```python
from build123d import *

# Parameters (mm, degrees)
SKETCH1_R           = 17.5
BOSS_EXTRUDE1_DEPTH = 3.5
CHAMFER1_SIZE       = 0.5
CUT_EXTRUDE1_DEPTH  = 1
SKETCH4_R           = 15.75
CUT_EXTRUDE2_DEPTH  = 1.5
FILLET1_R           = 1
THREAD1_PITCH       = 0.56


with BuildPart() as part:
    # Sketch1 → Boss-Extrude1 (new body)
    with BuildSketch(Plane(origin=(0, 0, 0), x_dir=(1, 0, 0), z_dir=(0, 1, 0))):
        with Locations(Location((0, 0, 0), (0, 0, 270))):
            Circle(SKETCH1_R)
    extrude(amount=BOSS_EXTRUDE1_DEPTH)

    # Chamfer1
    chamfer1_edges = [part.edges().sort_by_distance(p)[0] for p in [
        (0, 3.5, -17.5),
    ]]
    chamfer(chamfer1_edges, length=CHAMFER1_SIZE)

    # Sketch3 → Cut-Extrude1 (cut)
    with BuildSketch(Plane(origin=(0, 3.5, 0), x_dir=(1, 0, 0), z_dir=(0, 1, 0))):
        with BuildLine():
            Line((14.163644775, 9.216614608), (14.700580525, 9.526614608))
            ThreePointArc((14.700580525, 9.526614608), (15.170616014, 8.75875924), (15.600580525, 7.967768881))
            Line((15.600580525, 7.967768881), (15.063644775, 7.657768881))
            ThreePointArc((15.063644775, 7.657768881), (14.98776287, 7.647778839), (14.927042235, 7.694371422))
            Line((14.927042235, 7.694371422), (14.127042235, 9.080012068))
            ThreePointArc((14.127042235, 9.080012068), (14.117052192, 9.155893972), (14.163644775, 9.216614608))
        make_face()
        with BuildLine():
            Line((-0.8, 16.774383489), (0.8, 16.774383489))
            ThreePointArc((0.8, 16.774383489), (0.870710678, 16.803672811), (0.9, 16.874383489))
            Line((0.9, 16.874383489), (0.9, 17.494383489))
            ThreePointArc((0.9, 17.494383489), (0, 17.517518479), (-0.9, 17.494383489))
            Line((-0.9, 17.494383489), (-0.9, 16.874383489))
            ThreePointArc((-0.9, 16.874383489), (-0.870710678, 16.803672811), (-0.8, 16.774383489))
        make_face()
        with BuildLine():
            Line((15.063644775, -7.657768881), (15.600580525, -7.967768881))
            ThreePointArc((15.600580525, -7.967768881), (15.170616014, -8.75875924), (14.700580525, -9.526614608))
            Line((14.700580525, -9.526614608), (14.163644775, -9.216614608))
            ThreePointArc((14.163644775, -9.216614608), (14.117052192, -9.155893972), (14.127042235, -9.080012068))
            Line((14.127042235, -9.080012068), (14.927042235, -7.694371422))
            ThreePointArc((14.927042235, -7.694371422), (14.98776287, -7.647778839), (15.063644775, -7.657768881))
        make_face()
        with BuildLine():
            Line((0.9, -16.874383489), (0.9, -17.494383489))
            ThreePointArc((0.9, -17.494383489), (0, -17.517518479), (-0.9, -17.494383489))
            Line((-0.9, -17.494383489), (-0.9, -16.874383489))
            ThreePointArc((-0.9, -16.874383489), (-0.870710678, -16.803672811), (-0.8, -16.774383489))
            Line((-0.8, -16.774383489), (0.8, -16.774383489))
            ThreePointArc((0.8, -16.774383489), (0.870710678, -16.803672811), (0.9, -16.874383489))
        make_face()
        with BuildLine():
            Line((-14.163644775, -9.216614608), (-14.700580525, -9.526614608))
            ThreePointArc((-14.700580525, -9.526614608), (-15.170616014, -8.75875924), (-15.600580525, -7.967768881))
            Line((-15.600580525, -7.967768881), (-15.063644775, -7.657768881))
            ThreePointArc((-15.063644775, -7.657768881), (-14.98776287, -7.647778839), (-14.927042235, -7.694371422))
            Line((-14.927042235, -7.694371422), (-14.127042235, -9.080012068))
            ThreePointArc((-14.127042235, -9.080012068), (-14.117052192, -9.155893972), (-14.163644775, -9.216614608))
        make_face()
        with BuildLine():
            Line((-15.063644775, 7.657768881), (-15.600580525, 7.967768881))
            ThreePointArc((-15.600580525, 7.967768881), (-15.170616014, 8.75875924), (-14.700580525, 9.526614608))
            Line((-14.700580525, 9.526614608), (-14.163644775, 9.216614608))
            ThreePointArc((-14.163644775, 9.216614608), (-14.117052192, 9.155893972), (-14.127042235, 9.080012068))
            Line((-14.127042235, 9.080012068), (-14.927042235, 7.694371422))
            ThreePointArc((-14.927042235, 7.694371422), (-14.98776287, 7.647778839), (-15.063644775, 7.657768881))
        make_face()
    extrude(amount=-CUT_EXTRUDE1_DEPTH, mode=Mode.SUBTRACT)

    # Sketch4 → Cut-Extrude2 (cut)
    with BuildSketch(Plane(origin=(0, 0, 0), x_dir=(-1, 0, 0), z_dir=(0, -1, 0))):
        with Locations(Location((0, 0, 0), (0, 0, 90))):
            Circle(SKETCH4_R)
    extrude(amount=-CUT_EXTRUDE2_DEPTH, mode=Mode.SUBTRACT)

    # Fillet1
    fillet1_edges = [part.edges().sort_by_distance(p)[0] for p in [
        (0, 1.5, 15.75),
    ]]
    fillet(fillet1_edges, radius=FILLET1_R)

    # Thread1: the profile of Thread Profile2 profile screwed along a right-hand helix of 4 turns, 6 arcs to a turn; built about Z, then put on its axis
    thread1_z = Axis((0, 0, 0), (0, 0, 1))
    thread1_corners = [(17.5003, 0, -0.000173205), (17.5003, 0, 0.437673204), (17.229367062, 0, 0.281249999), (17.229367062, 0, 0.156249999)]
    with BuildLine(mode=Mode.PRIVATE) as thread1_profile:
        Line(thread1_corners[0], thread1_corners[1])
        Line(thread1_corners[1], thread1_corners[2])
        Line(thread1_corners[2], thread1_corners[3])
        Line(thread1_corners[3], thread1_corners[0])
    thread1_cap = Face(thread1_profile.wire())
    thread1_turn_angles = [0, 30, 60, 90, 120, 150, 180, 210, 240, 270, 300, 330, 360]
    thread1_turn_weights = [1, 0.8660254037844387, 1, 0.8660254037844387, 1, 0.8660254037844387, 1, 0.8660254037844387, 1, 0.8660254037844387, 1, 0.8660254037844387, 1]
    thread1_turn_rails = [Edge.make_bspline([Vector(p[0], p[1], 0).rotate(thread1_z, thread1_turn_angles[k]) / thread1_turn_weights[k] + Vector(0, 0, p[2] + THREAD1_PITCH * thread1_turn_angles[k] / 360) for k in range(13)], [0, 0, 0, 1, 1, 2, 2, 3, 3, 4, 4, 5, 5, 6, 6, 6], 2, thread1_turn_weights) for p in thread1_corners]
    thread1_turn_sides = [Face.make_surface_from_curves(thread1_turn_rails[p[0]], thread1_turn_rails[p[1]]) for p in [(0, 1), (1, 2), (2, 3), (3, 0)]]
    thread1 = Plane(origin=(0, 0, 0), x_dir=(1, 0, 0), z_dir=(0, 1, 0)) * Solid(Shell([*[p.moved(Location((0, 0, THREAD1_PITCH * i))) for i in range(4) for p in thread1_turn_sides], thread1_cap, thread1_cap.rotate(thread1_z, 1440).moved(Location((0, 0, THREAD1_PITCH * 1440 / 360)))]))
    add(thread1, mode=Mode.SUBTRACT)


solid = part.part
```
Input: part model. Units: mm. Frame: model coordinates. A direction names the side the tool comes from. Coordinates: 2 decimals unless noted, no trailing zeros. Write each question's results on one line, items separated by ' | '.
Item 1: Material intervals for probe 1 along Y at (x, z) = (4.5, 6); probe 2 along Z at (x, y) = (4, 1.25); probe 3 along Y at (x, z) = (15, -4.5), sorted ascending.
Conclusion:
probe 1: y = 1.5 to 3.5 | probe 2: z = -17.02 to -14.88, 14.88 to 16.76 | probe 3: y = 0.91 to 3.5
Item 2: Mould query, pull axis X, two halves, no side actions, for faces 1 (the flat face through (0, 1.5, 0)), 2 (the conical face through (-8.666, 3.365, 14.783)), 3 (the conical face through (8.666, 3.365, -14.783)). Classes: +X half, -X half, draft (parallel to the pull), parting line (faces both ways), or undercut.
Conclusion:
face 1: undercut | face 2: -X half | face 3: +X half
Item 3: Pin query (flat end, axial travel): pin 1 Ø2 at (x, y) = (-12, 2) entering from -Z; pin 2 Ø0.7 at (x, z) = (-15, 8.5) entering from +Y; pin 3 Ø1.5 at (x, y) = (-10.5, 3) entering from -Z. Return the tip coordinate at first contact, or that it passes through.
Conclusion:
pin 1: stops at z = -13.6 | pin 2: stops at y = 2.5 | pin 3: stops at z = -14.53
Item 4: Set-up query: faces 4 (the flat face through (-14.53, 3.01, 8.38)), 5 (the cylindrical face through (15.616, 0.246, 2.05)), 6 (the flat face through (0, 3, -16.774)). Return all of +Z, -Z, +X, -X, +Y, -Y with unobstructed straight access to the full face (end or side cutting, diameter ignored); none if empty.
Conclusion:
face 4: +Y | face 5: -Y | face 6: -Z, +Y
